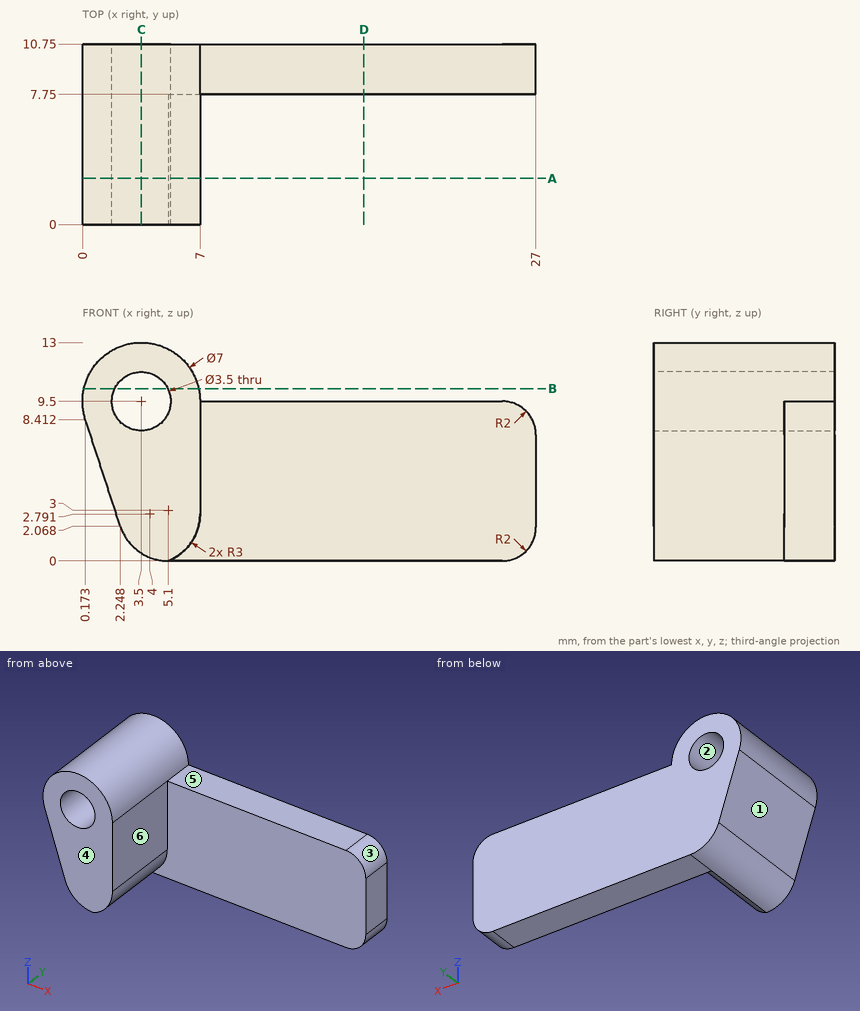
Input: dimensioned drawing with shaded views. Units: mm. Origin: part minimum x, y, z. A direction names the side the tool comes from. Round coordinates to 2 decimals unless told otherwise and drop trailing zeros. Order: outer loops, then holes, each group sorted by start corner. A loop starts at its lowest first (then second) coordinate and runs counter-clockwise, first axis right, second up. Notation, with made-up numbers: (63.5, -35.75) -> (120.5, -35.75) arc R34 ccw to (120.5, -1.75) -> close; hole circle Ø6 at (75.25, -38). An arc over 180 degrees is marked (long way). One line per item, written item: value. Start each with the question number.
Q1. Material intervals for probe 1 along Y at (x, z) = (16.25, 1); probe 2 along Z at (x, y) = (3.5, 7.5); probe 3 along Z at (x, y) = (20.75, 9.5), sorted ascending.
Q2. Pin query (flat end, axial travel): pin 1 (1.5 mm diameter, centred on y = 3, z = 11.5, fed in from -X); pin 2 (3 mm diameter, centred on x = 19, z = 6, fed in from -Y); pin 3 (2.5 mm diameter, centred on x = 16.5, y = 9, fed in from +Z). Return the tip coordinate at first contact, or that it passes through.
Q3. Section query D-D (x = 16.75). Return the cut outline in (y, z), plus the area to 3 significant figures.
Q4. Section query C-C (x = 3.5). Return the cut outline in (y, z).
Q5. Section query B-B (z = 10.25). Return the cut outline in (x, y).
Q6. Access query for the marked faces 4, 5 and 6. Directions: +Z, -Z, +X, -X, +Y, -Y. A direction counts if a zero-diameter tool reaches every point of the face in a straight line with its end or side. Return the directions, or none.
Q7. Draft query along Z for the marked faces 1, 2 and 3. Return one class per face: pulls with the +Z half, pulls with the -Z half, needs draft (parallel to the pull), parting line crosses it, or undercut.
Q8. Section query A-A (y = 2.75). Return the cut outline in (x, z).
Findings below:
1. probe 1: 7.75 to 10.75
1. probe 2: 0.46 to 7.75, 11.25 to 13
1. probe 3: 0 to 9.5
2. pin 1: x = 0.23
2. pin 2: y = 7.75
2. pin 3: z = 9.5
3. outline: (7.75, 0) -> (10.75, 0) -> (10.75, 9.5) -> (7.75, 9.5) -> close
3. area: 28.5 mm²
4. outline: (0, 0.46) -> (10.75, 0.46) -> (10.75, 7.75) -> (0, 7.75) -> close; (0, 11.25) -> (10.75, 11.25) -> (10.75, 13) -> (0, 13) -> close
5. outline: (0.08, 0) -> (1.92, 0) -> (1.92, 10.75) -> (0.08, 10.75) -> close; (5.08, 0) -> (6.92, 0) -> (6.92, 10.75) -> (5.08, 10.75) -> close
6. face 4: +Z, -Z, +X, -X, -Y
6. face 5: +Z, +X, +Y, -Y
6. face 6: +Z, -Z, +X, -Y
7. face 1: pulls with the -Z half
7. face 2: undercut
7. face 3: pulls with the +Z half
8. outline: (0.17, 8.41) -> (2.25, 2.07) arc R3 ccw to (5.1, 0) arc R3 ccw to (7, 2.79) -> (7, 9.5) arc R3.5 ccw (long way) to start; hole circle Ø3.5 at (3.5, 9.5)
